from build123d import *

# Parameters (mm, degrees)
ESBO_O1_W                                           = 100
ESBO_O1_H                                           = 40
RESSALTO_EXTRUS_O1_DEPTH                            = 10
RESSALTO_EXTRUS_O2_DEPTH                            = 10
ESBO_O3_R                                           = 3
CORTE_EXTRUS_O1_DEPTH                               = 74.484692283
REBAIXO_PARA_PARAFUSO_COM_CABE_A_PANELA_D           = 5.5
REBAIXO_PARA_PARAFUSO_COM_CABE_A_PANELA_CBORE_D     = 11
REBAIXO_PARA_PARAFUSO_COM_CABE_A_PANELA_CBORE_DEPTH = 3.7
ESBO_O6_W                                           = 40
ESBO_O6_H                                           = 5
CORTE_EXTRUS_O2_DEPTH                               = 88.749643874
FILETE1_R                                           = 5


with BuildPart() as part:
    # Esboço1 → Ressalto-extrusão1 (new body)
    with BuildSketch(Plane(origin=(0, 0, 0), x_dir=(1, 0, 0), z_dir=(0, 1, 0))):
        Rectangle(ESBO_O1_W, ESBO_O1_H)
    extrude(amount=RESSALTO_EXTRUS_O1_DEPTH)

    # Esboço2 → Ressalto-extrusão2 (add)
    with BuildSketch(Plane.XY.offset(20)):
        with BuildLine():
            Line((-20, 0), (-20, 40))
            ThreePointArc((-20, 40), (0, 60), (20, 40))
            Line((20, 40), (20, 0))
            Line((20, 0), (-20, 0))
        make_face()
    extrude(amount=-RESSALTO_EXTRUS_O2_DEPTH)

    # Esboço3 → Corte-extrusão1 (cut, through all)
    with BuildSketch(Plane(origin=(0, 10, 0), x_dir=(1, 0, 0), z_dir=(0, 1, 0))):
        with Locations(Location((-40, 10, 0), (0, 0, 270))):
            Circle(ESBO_O3_R)
        with Locations(Location((40, 10, 0), (0, 0, 270))):
            Circle(ESBO_O3_R)
    extrude(amount=-CORTE_EXTRUS_O1_DEPTH, mode=Mode.SUBTRACT)

    # Rebaixo para parafuso com cabeça panela de M51 (through all)
    with Locations(Plane(origin=(0, 40, 20), x_dir=(1, 0, 0), z_dir=(0, 0, 1))):
        with Locations((0, 0)):
            CounterBoreHole(REBAIXO_PARA_PARAFUSO_COM_CABE_A_PANELA_D / 2, REBAIXO_PARA_PARAFUSO_COM_CABE_A_PANELA_CBORE_D / 2, REBAIXO_PARA_PARAFUSO_COM_CABE_A_PANELA_CBORE_DEPTH)

    # Esboço6 → Corte-extrusão2 (cut, through all)
    with BuildSketch(Plane.XY.offset(20)):
        with Locations((0, 2.5)):
            Rectangle(ESBO_O6_W, ESBO_O6_H)
    extrude(amount=-CORTE_EXTRUS_O2_DEPTH, mode=Mode.SUBTRACT)

    # Filete1
    filete1_edges = [part.edges().sort_by_distance(p)[0] for p in [
        (-35, 10, 20),
        (35, 10, 20),
        (-20, 25, 10),
        (-20, 10, 15),
        (0, 60, 10),
        (20, 10, 15),
        (20, 25, 10),
        (0, 10, 10),
        (20, 25, 20),
        (0, 60, 20),
        (-20, 25, 20),
        (-20, 5, 0),
        (20, 5, 0),
        (0, 10, -20),
        (50, 5, 20),
        (-50, 5, 20),
    ]]
    fillet(filete1_edges, radius=FILETE1_R - 0.0001)  # a hair under: the kernel refuses the full size


solid = part.part
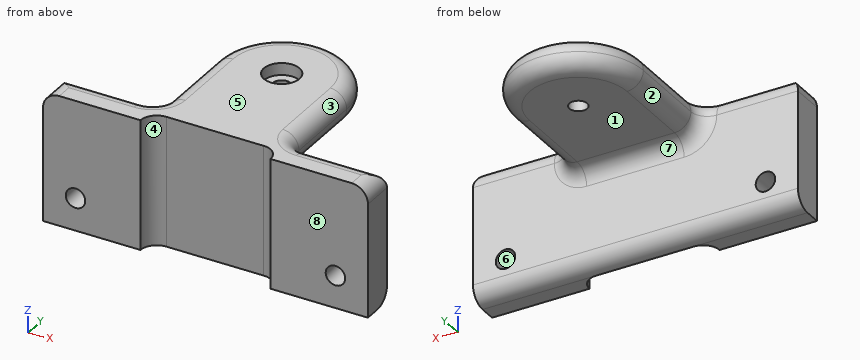
Design review of the part built by this model. Coordinates are the model's own, in mm. Face numbers are marked on the shaded views. A direction names the side the tool comes from. Give positions to 0.01 mm unless a question says otherwise; leave off trailing zeros. Write item = value, one per line. Start each with the question number.
Q1. Clearance check with flat-ended pins moving along their axes: pin 1 Ø15 at (x, z) = (4.5, 3) entering from -Y; pin 2 Ø9 at (x, y) = (0, 40) entering from -Z; pin 3 Ø10 at (x, z) = (3, -14.5) entering from +Y. State where each tip first meets the part, or that it passes through.
Q2. Mouldability with a two-part tool opening along Z and no side actions: class the marked faces 5, 6, 7 and 8 as released by +Z, released by -Z, zero draft, split by the parting line, or undercut.
Q3. We need section B-B on z = -10. State how many separate pieces and enclosed holes the cut face has, plus the area to 3 significant figures.
Q4. To check wall thickness, follow L1, parallel to X at y = 6, z = -10; L2, parallel to X at y = 2, z = -10; L3, parallel to Y at x = 13, z = -15. State the ranges of each line that lie inside material, in increasing order. Write a range as from..to.
Q5. Tool access review of the marked faces 1, 2, 3 and 4: name each direction out of +Z, -Z, +X, -X, +Y, -Y from which nothing blocks a thin tool from reaching the whole face with its end or side.
Working result:
q1.pin_1 = 5
q1.pin_2 = 10
q1.pin_3 = 10
q2.face_5 = released by +Z
q2.face_6 = undercut
q2.face_7 = released by -Z
q2.face_8 = zero draft
q3.separate_pieces = 3
q3.enclosed_holes = 0
q3.area = 691 mm²
q4.L1 = -50..-43, -37..37, 43..50
q4.L2 = -50..-43, -37..-19.58, 19.58..37, 43..50
q4.L3 = 5..10
q5.face_1 = -Z, +X, -X, +Y
q5.face_2 = -Z, -X, +Y
q5.face_3 = +Z, +X, +Y
q5.face_4 = +Z, -Z, -Y
